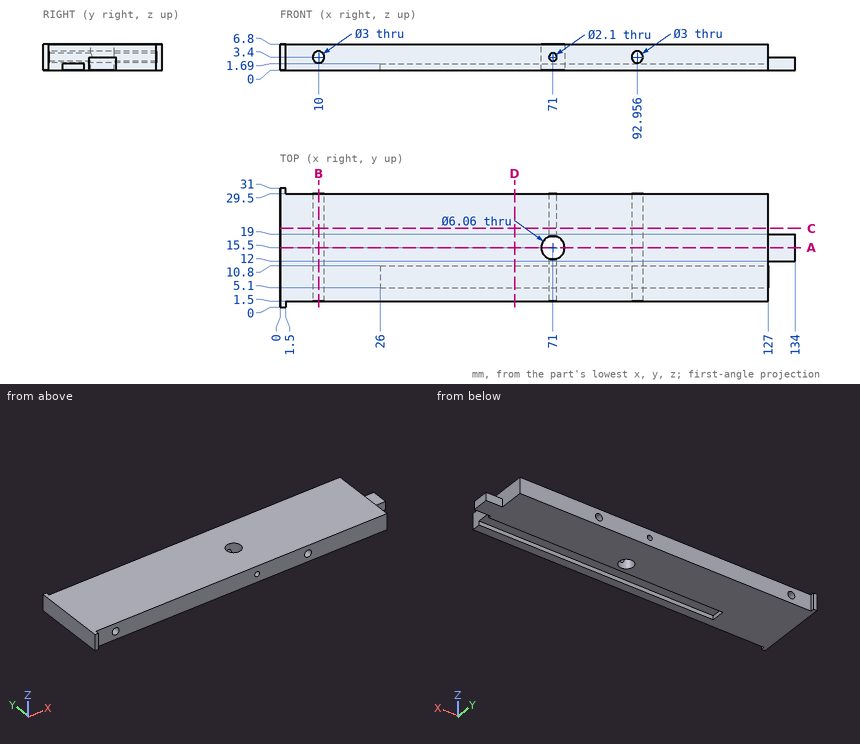
Input: dimensioned drawing with shaded views. Units: mm. Origin: part minimum x, y, z. Round coordinates to 2 decimals unless told otherwise and drop trailing zeros. Order: outer loops, then holes, each group sorted by start corner. A loop starts at its lowest first (then second) coordinate and runs counter-clockwise, first axis right, second up.
1. Cut plane B-B, the plane x = 10. Output: boundary loops of the cut face in (y, z), then the cut area to 3 significant figures.
The answers:
outline: (1.5, 0) - (29.5, 0) - (29.5, 1.9) - (1.5, 1.9) - close; (1.5, 4.9) - (29.5, 4.9) - (29.5, 6.8) - (1.5, 6.8) - close
area: 106 mm2
2. Material intervals for line 1 (X direction, y = 21, z = 3.5) (1 decimal); line 2 (Y direction, x = 78, z = 0.75); line 3 (X direction, y = 21, z = 6.25), sorted ascending.
The answers:
line 1: x = 0 to 8.5, 11.5 to 70, 72 to 91.5, 94.5 to 127
line 2: y = 1.5 to 5.1, 10.8 to 29.5
line 3: x = 0 to 127
3. Cut plane C-C, the plane y = 20.5. Output: boundary loops of the cut face in (x, z), then the cut area to 3 significant figures.
The answers:
outline: (0, 0) - (127, 0) - (127, 6.8) - (0, 6.8) - close; hole circle Ø3 at (10, 3.4); hole circle Ø2.1 at (71, 3.4); hole circle Ø3 at (92.96, 3.4)
area: 846 mm2
4. Cut plane D-D, the plane x = 61. Output: boundary loops of the cut face in (y, z).
The answers:
outline: (1.5, 0) - (5.1, 0) - (5.1, 1.69) - (10.8, 1.69) - (10.8, 0) - (29.5, 0) - (29.5, 6.8) - (1.5, 6.8) - close
5. Pin query (flat end, axial travel): P1, Ø2, axis at y = 17.5, z = 3.5, coming from the +X side; P2, Ø1, axis at x = 130.5, z = 2, coming from the +Y side; P3, Ø0.5, axis at x = 86.5, z = 0.5, coming from the +Y side; P4, Ø4, axis at y = 5, z = 3, coming from the +X side. Return the tip coordinate at first contact, or that it passes through.
The answers:
P1: stops at x = 134
P2: stops at y = 19
P3: stops at y = 29.5
P4: stops at x = 127
6. Cut plane A-A, the plane y = 15.5. Output: boundary loops of the cut face in (x, z), then the cut area to 3 significant figures.
The answers:
outline: (0, 0) - (67.97, 0) - (67.97, 6.8) - (0, 6.8) - close; (74.03, 0) - (134, 0) - (134, 3.4) - (127, 3.4) - (127, 6.8) - (74.03, 6.8) - close; hole circle Ø3 at (10, 3.4); hole circle Ø3 at (92.96, 3.4)
area: 832 mm2
